```python
from build123d import *

# Parameters (mm, degrees)
F0_W      = 60
F0_H      = 40
F1_DEPTH  = 40
F2_W      = 20
F2_H      = 10
F3_DEPTH  = 10
F4_DEPTH  = 30
F5_W      = 60
F5_H      = 10
F6_DEPTH  = 10
F7_W      = 40
F7_H      = 20
F8_DEPTH  = 10
F10_DEPTH = 10
F11_W     = 20
F11_H     = 10
F12_DEPTH = 10
F14_DEPTH = 10


with BuildPart() as f1:
    # F0 (on Top) → F1 (new body)
    with BuildSketch(Plane.XY):
        with Locations((30, 20)):
            Rectangle(F0_W, F0_H)
    extrude(amount=F1_DEPTH)

    # F2 (on face) → F3 (cut)
    with BuildSketch(Plane.XY.offset(40)):
        with Locations((10, 35)):
            Rectangle(F2_W, F2_H)
    extrude(amount=-F3_DEPTH, mode=Mode.SUBTRACT)

    # F2 (on face) → F4 (cut)
    with BuildSketch(Plane.XY.offset(40)):
        Polygon((20, 30), (0, 30), (0, 10), (60, 10), (60, 30), align=None)
    extrude(amount=-F4_DEPTH, mode=Mode.SUBTRACT)

    # F5 (on face) → F6 (cut)
    with BuildSketch(Plane.XZ):
        with Locations((30, 35)):
            Rectangle(F5_W, F5_H)
    extrude(amount=-F6_DEPTH, mode=Mode.SUBTRACT)

    # F7 (on face) → F8 (cut)
    with BuildSketch(Plane.XZ):
        with Locations((40, 20)):
            Rectangle(F7_W, F7_H)
    extrude(amount=-F8_DEPTH, mode=Mode.SUBTRACT)

    # F9 (on face) → F10 (cut)
    with BuildSketch(Plane.XZ):
        with BuildLine():
            ThreePointArc((10, 30), (12.9289321881, 22.9289321881), (20, 20))
            Line((20, 20), (20, 30))
            Line((20, 30), (10, 30))
        make_face()
    extrude(amount=-F10_DEPTH, mode=Mode.SUBTRACT)

    # F11 (on face) → F12 (cut)
    with BuildSketch(Plane(origin=(0, 40, 0), x_dir=(-1, 0, 0), z_dir=(0, 1, 0))):
        with Locations((-10, 25)):
            Rectangle(F11_W, F11_H)
    extrude(amount=-F12_DEPTH, mode=Mode.SUBTRACT)

    # F13 (on face) → F14 (cut)
    with BuildSketch(Plane.XZ.offset(-30)):
        with BuildLine():
            Line((40, 20), (50, 20))
            ThreePointArc((50, 20), (40, 30), (30, 20))
            Line((30, 20), (40, 20))
        make_face()
        with BuildLine():
            ThreePointArc((30, 20), (32.9289321881, 12.9289321881), (40, 10))
            ThreePointArc((40, 10), (47.0710678119, 12.9289321881), (50, 20))
            Line((50, 20), (40, 20))
            Line((40, 20), (30, 20))
        make_face()
        with BuildLine():
            ThreePointArc((40, 40), (54.1421356237, 34.1421356237), (60, 20))
            Line((60, 20), (60, 40))
            Line((60, 40), (40, 40))
        make_face()
        with BuildLine():
            ThreePointArc((20, 20), (25.8578643763, 34.1421356237), (40, 40))
            Line((40, 40), (20, 40))
            Line((20, 40), (20, 20))
        make_face()
    extrude(amount=-F14_DEPTH, mode=Mode.SUBTRACT)


solid = f1.part
```
CAD build for the part. Positions are in the model's coordinates, mm. A direction names the side the tool comes from. Round coordinates to 2 decimals unless told otherwise and drop trailing zeros. Write each loop counter-clockwise with the first axis right and the second up, starting at its lowest first coordinate (ties: lowest second). Pieces come first, ordered by that corner, then holes. Notation, with made-up numbers: M 16.25,23.5 L 40.25,23.5 A7 cw 40.25,36.5 Z; hole C -26.5,-19 d5. An arc over 180 degrees is marked long. One line per question, with ' | ' between items.
1. Cut at D-D on y = 33. Write the cut outline in (x, z), and give its area (3 significant figures).
Working result:
outline: M 0,0 L 60,0 L 60,20 A20 ccw 20,20 L 0,20 Z; hole C 40,20 d20 | area: 1,510 mm2
2. Cut at B-B on y = 9. Write the cut outline in (x, z), and give its area (3 significant figures).
Working result:
outline: M 0,0 L 60,0 L 60,10 L 20,10 L 20,20 A10 cw 10,30 L 0,30 Z | area: 921 mm2
3. Probe L1, parallel to Y at x = 6.5, z = 11; L2, parallel to Y at x = 34.5, z = 34.5; L3, parallel to Z at x = 46, y = 12. List the from-to ranges inside material, lowest first. Write a range as from..to.
Working result:
L1: 0..10, 30..40 | L2: 30..40 | L3: 0..10
4. Mould opens along Y. For faces 4 (the flat face through (30, 15, 10)), 5 (the flat face through (30, 20, 0)), 6 (the flat face through (23, 0, 8)), 7 (the flat face through (30, 30, 25)) say: pulls with the +Y half, pulls with the -Y half, needs draft (parallel to the pull), parting line crosses it, or undercut.
Working result:
face 4: undercut | face 5: needs draft | face 6: pulls with the -Y half | face 7: undercut
5. Which spindle directions (+Z, -Z, +X, -X, +Y, -Y) get a long thin tool onto all of the face, cutting with end or side? Do faces 1 (the flat face through (8, 10, 18)), 2 (the flat face through (10, 35, 20)), 3 (the flat face through (20, 5, 15)). Say none if no direction does.
Working result:
face 1: +Z, +X, -X | face 2: +Z, -X, +Y | face 3: +Z, +X, -Y
6. Pin check, flat tips, straight feed: pin 1 Ø5 at (x, y) = (16.5, 29) entering from +Z; pin 2 Ø2 at (x, y) = (51, 7) entering from +Z; pin 3 Ø5 at (y, z) = (34.5, 27) entering from +X. Stop position of each tip, or through.
Working result:
pin 1: z = 20 | pin 2: z = 10 | pin 3: x = 59.49
7. Cut at C-C on x = 8. Write the cut outline in (y, z), and give its area (3 significant figures).
Working result:
outline: M 0,0 L 40,0 L 40,20 L 30,20 L 30,10 L 10,10 L 10,30 L 0,30 Z | area: 700 mm2
8. Cut at A-A on z = 12. Write the cut outline in (x, y).
Working result:
outline: M 0,0 L 20,0 L 20,10 L 0,10 Z; M 0,30 L 34,30 L 34,40 L 0,40 Z; M 46,30 L 60,30 L 60,40 L 46,40 Z
